Work out the finished part from the listing and answer in its coordinate system (mm). A direction names the side the tool comes from. Give positions to 0.01 mm unless a question says otherwise; leave off trailing zeros. Order: outer loops, then holes, each group sorted by start corner. A loop starts at its lowest first (then second) coordinate and runs counter-clockwise, first axis right, second up. Notation, with made-up numbers: (-27, 5) -> (10, 5) arc R22 cw to (10, 27) -> close; hole circle Ø3 at (-29, 27). An arc over 180 degrees is marked (long way). Answer as CSV lines item,"result". Start each with the question number.
1. A cutting plane is placed at A-A (x = 0). Give the vertices of the cut face in (y, z).
2. For faces 4 (the flat face through (2, -0.477, 2)), 5 (the flat face through (1.95, -5, 2)), 6 (the flat face through (-1.65, -2, 2)), 7 (the flat face through (-0.15, -3, 2)), 8 (the flat face through (2, 5, 2)), determine the directions among +Z, -Z, +X, -X, +Y, -Y from which every point of the face is accessible in a straight line to the end or side of a thin tool.
3. A cutting plane is placed at D-D (y = 8.5). Give the vertices of the cut face in (x, z), then the cut area to 3 significant figures.
4. A cutting plane is placed at C-C (z = 2). Give the vertices of the cut face in (x, y), then the cut area to 3 significant figures.
5. For a pull along X with two mould halves and no side action, classify faces 1 (the flat face through (0, 3.315, 2)), 2 (the flat face through (3.244, 3, 2)), 3 (the flat face through (-1.95, -5, 2)) as released by +X, released by -X, zero draft, split by the parting line, or undercut.
6. A cutting plane is placed at B-B (y = 0). Give the vertices of the cut face in (x, z).
7. Flat-ended cylindrical pins translate along their axes: pin 1 (1 mm diameter, centred on y = -2.5, z = 2, fed in from +X); pin 2 (1.3 mm diameter, centred on y = -4.5, z = 1.5, fed in from +X); pin 3 (1.6 mm diameter, centred on x = -1, z = 1.5, fed in from +Y). Find the tip coordinate at first contact, or state that the pin passes through.
8. Find the intervals of material crossed by L1, parallel to X at y = 0, z = 1.55; L2, parallel to X at y = -4, z = 1; L3, parallel to Y at x = 0.25, z = 2.15, in increasing order.
from build123d import *

# Parameters (mm, degrees)
SALIENTE_EXTRUIR2_DEPTH = 3.3


with BuildPart() as part:
    # Croquis2 → Saliente-Extruir2 (new body)
    with BuildSketch(Plane.XY):
        with BuildLine():
            Line((-0.15, -3.776969601), (-0.15, -0.476969601))
            ThreePointArc((-0.15, -0.476969601), (0, 0.5), (0.15, -0.476969601))
            Line((0.15, -0.476969601), (0.15, -3.776969601))
            Line((0.15, -3.776969601), (0.15, -5.384848335))
            Line((0.15, -5.384848335), (1.95, -5.384848335))
            Line((1.95, -5.384848335), (1.95, -3.776969601))
            Line((1.95, -3.776969601), (1.65, -3.776969601))
            Line((1.65, -3.776969601), (1.65, -0.476969601))
            Line((1.65, -0.476969601), (3.24401575, -0.476969601))
            Line((3.24401575, -0.476969601), (3.24401575, 1.350254565))
            Line((3.24401575, 1.350254565), (3.24401575, 6.615151665))
            ThreePointArc((3.24401575, 6.615151665), (0, 9.859167415), (-3.24401575, 6.615151665))
            Line((-3.24401575, 6.615151665), (-3.24401575, 1.350254565))
            Line((-3.24401575, 1.350254565), (-3.24401575, -0.476969601))
            Line((-3.24401575, -0.476969601), (-1.65, -0.476969601))
            Line((-1.65, -0.476969601), (-1.65, -3.776969601))
            Line((-1.65, -3.776969601), (-1.95, -3.776969601))
            Line((-1.95, -3.776969601), (-1.95, -5.384848335))
            Line((-1.95, -5.384848335), (-0.15, -5.384848335))
            Line((-0.15, -5.384848335), (-0.15, -3.776969601))
        make_face()
        Polygon((-2, 6.615151665), (0, 6.615151665), (2, 6.615151665), (2, 3.315151665), (-2, 3.315151665), align=None, mode=Mode.SUBTRACT)
    extrude(amount=SALIENTE_EXTRUIR2_DEPTH)


solid = part.part
Answer sheet:
1,outline,"(0.5, 0) -> (3.32, 0) -> (3.32, 3.3) -> (0.5, 3.3) -> close; (6.62, 0) -> (9.86, 0) -> (9.86, 3.3) -> (6.62, 3.3) -> close"
2,face 4,"+Z, -Z, +X"
2,face 5,"+Z, -Z, +X, -Y"
2,face 6,"+Z, -Z, -X"
2,face 7,"+Z, -Z, -Y"
2,face 8,"+Z, -Z"
3,outline,"(-2.64, 0) -> (2.64, 0) -> (2.64, 3.3) -> (-2.64, 3.3) -> close"
3,area,"17.4 mm^2"
4,outline,"(-3.24, -0.48) -> (-1.65, -0.48) -> (-1.65, -3.78) -> (-1.95, -3.78) -> (-1.95, -5.38) -> (-0.15, -5.38) -> (-0.15, -0.48) arc R0.5 cw (long way) to (0.15, -0.48) -> (0.15, -5.38) -> (1.95, -5.38) -> (1.95, -3.78) -> (1.65, -3.78) -> (1.65, -0.48) -> (3.24, -0.48) -> (3.24, 6.62) arc R3.24 ccw to (-3.24, 6.62) -> close; hole (-2, 3.32) -> (2, 3.32) -> (2, 6.62) -> (-2, 6.62) -> close"
4,area,"64.3 mm^2"
5,face 1,"undercut"
5,face 2,"released by +X"
5,face 3,"released by -X"
6,outline,"(-3.24, 0) -> (-0.5, 0) -> (-0.5, 3.3) -> (-3.24, 3.3) -> close; (0.5, 0) -> (3.24, 0) -> (3.24, 3.3) -> (0.5, 3.3) -> close"
7,pin 1,"stops at x = 1.65"
7,pin 2,"stops at x = 1.95"
7,pin 3,"stops at y = 9.85"
8,L1,"x = -3.24 to -0.5, 0.5 to 3.24"
8,L2,"x = -1.95 to -0.15, 0.15 to 1.95"
8,L3,"y = -5.38 to -0.43, 0.43 to 3.32, 6.62 to 9.85"
